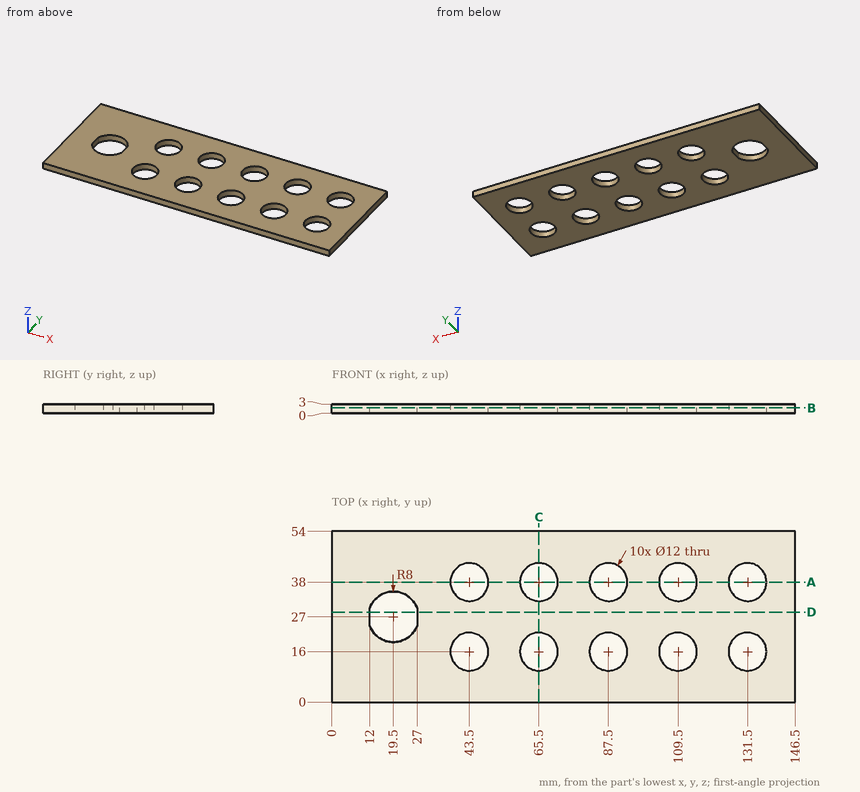
Part print with two shaded views. Sizes in mm from the minimum x, y, z corner. Give positions to 0.01 mm unless a question says otherwise; leave off trailing zeros. Order: outer loops, then holes, each group sorted by start corner. A loop starts at its lowest first (then second) coordinate and runs counter-clockwise, first axis right, second up.
(1) Flat gauge pin, fed straight in: pin 1 (11 mm diameter, centred on x = 131.5, y = 38, fed in from +Z). Where does the tip first touch, or does it go through?
(2) Drill centre lines: L1, parallel to Y at x = 43.5, z = 2.45; L2, parallel to X at y = 28.5, z = 0.5; L3, parallel to X at y = 15, z = 2.05. Where is each one in solid material? Low to high.
(3) Saw through at D-D, the plane y = 28.5. Give the cut face in (x, z), then the cut area to 4 significant figures.
(4) Saw through at B-B, the plane z = 1.8. State how many separate pieces and enclosed holes the cut face has, then the cut area to 3 significant figures.
(5) Saw through at C-C, the plane x = 65.5. Give the cut face in (y, z).
(6) Saw through at A-A, the plane y = 38. Give the cut face in (x, z), then the cut area to 4 significant figures.
Results found:
1. pin 1: passes through
2. L1: y = 0 to 10, 22 to 32, 44 to 54
2. L2: x = 0 to 12, 27 to 146.5
2. L3: x = 0 to 37.58, 49.42 to 59.58, 71.42 to 81.58, 93.42 to 103.58, 115.42 to 125.58, 137.42 to 146.5
3. outline: (0, 0) - (12, 0) - (12, 3) - (0, 3) - close; (27, 0) - (146.5, 0) - (146.5, 3) - (27, 3) - close
3. area: 394.5 mm2
4. separate pieces: 1
4. enclosed holes: 11
4. area: 6,580 mm2
5. outline: (0, 0) - (10, 0) - (10, 3) - (0, 3) - close; (22, 0) - (32, 0) - (32, 3) - (22, 3) - close; (44, 0) - (54, 0) - (54, 3) - (44, 3) - close
6. outline: (0, 0) - (37.5, 0) - (37.5, 3) - (0, 3) - close; (49.5, 0) - (59.5, 0) - (59.5, 3) - (49.5, 3) - close; (71.5, 0) - (81.5, 0) - (81.5, 3) - (71.5, 3) - close; (93.5, 0) - (103.5, 0) - (103.5, 3) - (93.5, 3) - close; (115.5, 0) - (125.5, 0) - (125.5, 3) - (115.5, 3) - close; (137.5, 0) - (146.5, 0) - (146.5, 3) - (137.5, 3) - close
6. area: 259.5 mm2
